from build123d import *

# Parameters (mm, degrees)
F0_R      = 28.575
F1_DEPTH  = 20.32
F2_R      = 27.305
F3_DEPTH  = 17.78
F4_R      = 1.733709
F5_DEPTH  = 28.576
F6_R      = 1.562885
F7_DEPTH  = 28.481089
F8_R      = 41.275
F9_DEPTH  = 2.54
F10_R     = 27.305
F11_DEPTH = 2.54
F12_R     = 2.54
F13_DEPTH = 22.861
F14_R     = 2.54
F15_DEPTH = 22.861
F16_R     = 2.54
F17_DEPTH = 22.861
F18_R     = 2.54
F19_DEPTH = 22.861


with BuildPart() as f1:
    # F0 (on Top) → F1 (new body)
    with BuildSketch(Plane.XY):
        with Locations((0, -0.094911)):
            Circle(F0_R)
    extrude(amount=F1_DEPTH)

    # F2 (on face) → F3 (cut)
    with BuildSketch(Plane.XY.offset(20.32)):
        Circle(F2_R)
    extrude(amount=-F3_DEPTH, mode=Mode.SUBTRACT)

    # F4 (on Right) → F5 (cut, through all)
    with BuildSketch(Plane.YZ):
        with Locations((-10.845167, 10.345303)):
            Circle(F4_R)
    extrude(amount=F5_DEPTH, mode=Mode.SUBTRACT)

    # F6 (on Front) → F7 (cut, through all)
    with BuildSketch(Plane.XZ):
        with Locations((11.812109, 10.026056)):
            Circle(F6_R)
    extrude(amount=-F7_DEPTH, mode=Mode.SUBTRACT)

    # F8 (on face) → F9 (join)
    with BuildSketch(Plane.XY.offset(20.32)):
        Circle(F8_R)
    extrude(amount=F9_DEPTH)

    # F10 (on face) → F11 (cut)
    with BuildSketch(Plane.XY.offset(22.86)):
        Circle(F10_R)
    extrude(amount=-F11_DEPTH, mode=Mode.SUBTRACT)

    # F12 (on Top) → F13 (cut, through all)
    with BuildSketch(Plane.XY):
        with Locations((0, 34.925)):
            Circle(F12_R)
    extrude(amount=F13_DEPTH, mode=Mode.SUBTRACT)

    # F14 (on face) → F15 (cut, through all)
    with BuildSketch(Plane.XY.offset(22.86)):
        with Locations((-34.925, 0)):
            Circle(F14_R)
    extrude(amount=-F15_DEPTH, mode=Mode.SUBTRACT)

    # F16 (on face) → F17 (cut, through all)
    with BuildSketch(Plane.XY.offset(22.86)):
        with Locations((0, -34.925)):
            Circle(F16_R)
    extrude(amount=-F17_DEPTH, mode=Mode.SUBTRACT)

    # F18 (on face) → F19 (cut, through all)
    with BuildSketch(Plane.XY.offset(22.86)):
        with Locations((34.925, 0)):
            Circle(F18_R)
    extrude(amount=-F19_DEPTH, mode=Mode.SUBTRACT)


solid = f1.part
The listing builds one solid part. Answer for the finished solid, in the listing's coordinates (mm). A direction names the side the tool comes from. Coordinates: 2 decimals unless noted, no trailing zeros. Write each loop counter-clockwise with the first axis right and the second up, starting at its lowest first coordinate (ties: lowest second). Pieces come first, ordered by that corner, then holes. Notation, with made-up numbers: (72.25, 57.25) - (109.25, 57.25) arc R16 cw to (109.25, 88.25) - close; hole circle Ø5 at (-39, 38). An arc over 180 degrees is marked (long way). Put each result on its own line as item: value.
1. The part is cut by section A-A on x = 0. Give the vertices of the cut face in (y, z) (3 decimals).
Answer sheet:
outline: (-41.275, 20.32) - (-37.465, 20.32) - (-37.465, 22.86) - (-41.275, 22.86) - close; (-32.385, 20.32) - (-28.67, 20.32) - (-28.67, 0) - (28.48, 0) - (28.48, 20.32) - (32.385, 20.32) - (32.385, 22.86) - (27.305, 22.86) - (27.305, 2.54) - (-27.305, 2.54) - (-27.305, 22.86) - (-32.385, 22.86) - close; (37.465, 20.32) - (41.275, 20.32) - (41.275, 22.86) - (37.465, 22.86) - close
2. Flat-ended cylindrical pins translate along their axes: pin 1 Ø4 at (x, z) = (11.81, 10.03) entering from +Y; pin 2 Ø4 at (y, z) = (-10.85, 10.35) entering from -X; pin 3 Ø8 at (x, y) = (34.925, 0) entering from +Z; pin 4 Ø8 at (x, z) = (-5.5, 5) entering from -Y. Find the tip coordinate at first contact, or state that the pin passes through.
Answer sheet:
pin 1: stops at y = 26.74
pin 2: stops at x = -27.2
pin 3: stops at z = 22.86
pin 4: stops at y = -28.63
3. A tool of negligible diameter and unlimited length cuts with its end or side. For faces 4 (the face through (-28.547, 1.161, 10.018)), 5 (the face through (1.365, -32.783, 21.608)), 6 (the face through (12.652, 25.178, 11.344)), 7 (the face through (-20.125, 18.454, 12.842)), from which of +Z, -Z, +X, -X, +Y, -Y can it reach the whole face along a straight path? Write none if from no direction.
Answer sheet:
face 4: -Z
face 5: +Z, -Z
face 6: +Y
face 7: +Z
4. Find the intervals of material crossed by line 1 along Y through (x, z) = (0, 20.9) (3 decimals); line 2 along Z through (x, y) = (-11.5, -38); line 3 along X through (y, z) = (19.5, 15.5), in increasing order. Write a range as from..to.
Answer sheet:
line 1: y = -41.275..-37.465, -32.385..-27.305, 27.305..32.385, 37.465..41.275
line 2: z = 20.32..22.86
line 3: x = -20.8..-19.11, 19.11..20.8
5. The part is cut by section C-C on y = 22. Give the vertices of the cut face in (x, z), plus the area to 3 significant figures.
Answer sheet:
outline: (-34.92, 20.32) - (-18.12, 20.32) - (-18.12, 0) - (18.12, 0) - (18.12, 20.32) - (34.92, 20.32) - (34.92, 22.86) - (16.17, 22.86) - (16.17, 2.54) - (-16.17, 2.54) - (-16.17, 22.86) - (-34.92, 22.86) - close
area: 257 mm^2
6. The part is cut by section B-B on x = -26. Give the vertices of the cut face in (y, z), plus the area to 3 significant figures.
Answer sheet:
outline: (-32.06, 20.32) - (-11.95, 20.32) - (-11.95, 0) - (11.76, 0) - (11.76, 20.32) - (32.06, 20.32) - (32.06, 22.86) - (8.34, 22.86) - (8.34, 2.54) - (-8.34, 2.54) - (-8.34, 22.86) - (-32.06, 22.86) - close
area: 306 mm^2
7. The part is cut by section D-D on z = 7.25. Give the vertices of the cut face in (x, y) (3 decimals).
Answer sheet:
outline: circle Ø57.15 at (0, -0.095); hole circle Ø54.61 at (0, 0)
8. Determine the mould class of faces 1 (the face through (0, 0, 0)), 2 (the face through (9, -27, 22.86)), 3 (the face through (25.65, -12.12, 11.52)) for opening direction Z: pulls with the +Z half, pulls with the -Z half, needs draft (parallel to the pull), parting line crosses it, or undercut.
Answer sheet:
face 1: pulls with the -Z half
face 2: pulls with the +Z half
face 3: undercut
